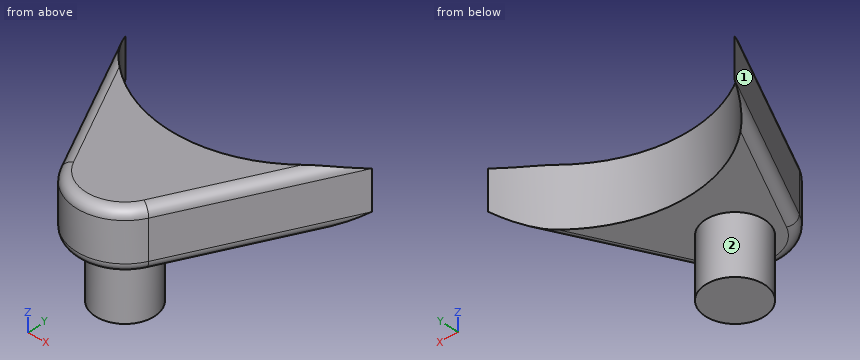
Autodesk Inventor part; units mm, degrees
ref_plane "YZ Plane" through (0, 0, 0) normal (1, 0, 0) x (0, 1, 0)
ref_plane "XZ Plane" through (0, 0, 0) normal (0, 1, 0) x (-1, 0, 0)
ref_plane "XY Plane" through (0, 0, 0) normal (0, 0, 1) x (1, 0, 0)
sketch "Sketch1" plane through (0, 0, 0) normal (0, 0, 1) x (1, 0, 0)
  circle A0 centre (0, 0) radius 7
  circle A1 centre (0, -10) radius 1.5
  circle A2 centre (0, -10) radius 2.5
  line L0 (0, -16.4) -> (0, 10.9)
  line L1 (-2.2326, -11.125) -> (-6.2512, -3.15)
  line L2 (2.2326, -11.125) -> (6.2512, -3.15)
  dimension "d0" = 14
  dimension "d1" = 3
  dimension "d2" = 1
  dimension "d3" = 10
extrude "Extrusion1" add sketch "Sketch1" along normal blind 3 contours L2 A2 L0 A0 | L0 A2 L1 A0 | A2 L0 A1 | L0 A1 A2 | L0 A1 | A1 L0
extrude "Extrusion2" add sketch "Sketch1" against normal blind 3 contours L0 A1 | A1 L0
fillet "Fillet1" radius 0.5 6 edges at (0, -12.5, 3) (-4.2419, -7.1375, 3) (4.2419, -7.1375, 3) (0, -12.5, 0) (-4.2419, -7.1375, 0) (4.2419, -7.1375, 0)
properties part number "Joystick Extra Hook"
Can you work these out from the model? Positions are in its coordinate system, mm. Face numbers are marked on the shaded views. A direction names the side the tool comes from. Coordinates: 2 decimals unless noted, no trailing zeros. Order: outer loops, then holes, each group sorted by start corner. A loop starts at its lowest first (then second) coordinate and runs counter-clockwise, first axis right, second up. Notation, with made-up numbers: (51.5, 10) - (58.5, 10) arc R14 cw to (58.5, 19) - close; hole circle Ø5 at (41, 47). An arc over 180 degrees is marked (long way). Answer in a Markdown table with one row per item.
1. Suppose I cut it at C-C (z = -0.75). Please give me the cut outline in (x, y), and give its area (3 significant figures).
Reply:
| item | result |
|---|---|
| outline | circle Ø3 at (0, -10) |
| area | 7.07 mm^2 |
2. For pin 1 (1.5 mm diameter, centred on y = -10, z = 1, fed in from -X); pin 2 (2 mm diameter, centred on x = -1, z = -2, fed in from -Y); pin 3 (2 mm diameter, centred on y = -9, z = -2, fed in from +X), each with a flat end and sliding along its axis, tell me the tip position at first contact or that it passes through.
Reply:
| item | result |
|---|---|
| pin 1 | stops at x = -3.18 |
| pin 2 | stops at y = -11.5 |
| pin 3 | stops at x = 1.5 |
3. Suppose I cut it at D-D (z = 2.75). Please give me the cut outline in (x, y).
Reply:
| item | result |
|---|---|
| outline | (-5.76, -3.98) - (-2.17, -11.09) arc R2.43 ccw to (2.17, -11.09) - (5.76, -3.98) arc R7 cw to start |
4. Suppose I cut it at A-A (x = 0). Please give me the cut outline in (y, z), and give its area (3 significant figures).
Reply:
| item | result |
|---|---|
| outline | (-12.5, 0.5) arc R0.5 ccw to (-12, 0) - (-11.5, 0) - (-11.5, -3) - (-8.5, -3) - (-8.5, 0) - (-7, 0) - (-7, 3) - (-12, 3) arc R0.5 ccw to (-12.5, 2.5) - close |
| area | 25.4 mm^2 |
5. If I drill on line 1 along Z through (x, y) = (1.5, -11); line 2 along X through (y, z) = (-10.75, 2.5); line 3 along Z through (x, y) = (-2, -11), over which ranges is the centre line in solid material (lowest first)?
Reply:
| item | result |
|---|---|
| line 1 | z = 0 to 3 |
| line 2 | x = -2.42 to 2.42 |
| line 3 | z = 0.06 to 2.94 |
6. Suppose I cut it at B-B (z = 1.5). Please give me the cut outline in (x, y) (3 decimals), and give its area (3 significant figures).
Reply:
| item | result |
|---|---|
| outline | (-6.251, -3.15) - (-2.233, -11.125) arc R2.5 ccw to (2.233, -11.125) - (6.251, -3.15) arc R7 cw to start |
| area | 37.6 mm^2 |
7. For the marked faces 1 and 2, which set-ups out of +Z, -Z, +X, -X, +Y, -Y let a thin tool reach every point of the face, with its end or its side?
Reply:
| item | result |
|---|---|
| face 1 | +Z, -Z, -X, -Y |
| face 2 | -Z |
